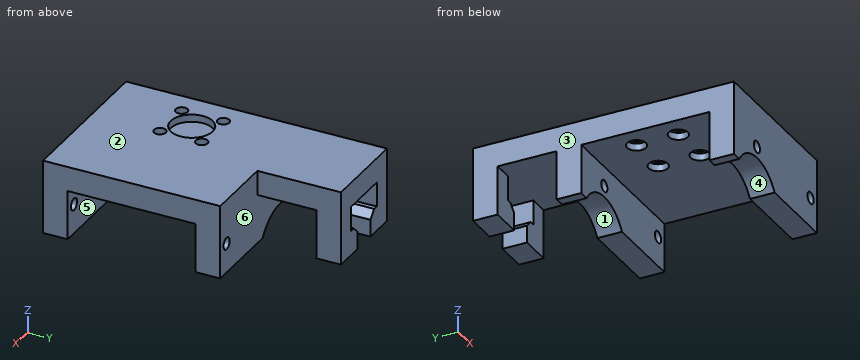
```python
from build123d import *

# Parameters (mm, degrees)
SKETCH_1_W                   = 32.5
SKETCH_1_H                   = 36
EXTRUDE_1_DEPTH              = 15
SKETCH_2_W                   = 10
SKETCH_2_H                   = 26
CUT_EXTRUDE_1_DEPTH          = 41.065571255
HOLE_WIZARD_M2_1_D           = 2.4
HOLE_WIZARD_M2_1_DEPTH       = 5
CUT_EXTRUDE_3_DEPTH          = 39.079686186
CUT_EXTRUDE_3_DEPTH_BACK     = 39.079686186
SKETCH_4_R                   = 8.25
SKETCH_4_R_2                 = 1.2
HOLE_WIZARD_M2_2_D           = 2.4
HOLE_WIZARD_M2_2_CBORE_D     = 3.85
HOLE_WIZARD_M2_2_CBORE_DEPTH = 1.45
SKETCH_13_W                  = 18
SKETCH_13_H                  = 15
EXTRUDE_3_DEPTH              = 17
CUT_EXTRUDE_4_DEPTH          = 42.401237904
CUT_EXTRUDE_4_DEPTH_BACK     = 10
SKETCH_14_W                  = 18
SKETCH_14_H                  = 12
CUT_EXTRUDE_5_REACH          = 59.429
SKETCH_15_W                  = 5
SKETCH_15_H                  = 10
CUT_EXTRUDE_START            = -5
SKETCH_16_W                  = 10
SKETCH_16_H                  = 5
CUT_EXTRUDE_6_DEPTH          = 5
CHAMFER_1_SIZE               = 1.5
CUT_EXTRUDE_7_DEPTH          = 1.5


with BuildPart() as part:
    # ｽｹｯﾁ1 → ﾎﾞｽ - 押し出し1 (new body)
    with BuildSketch(Plane.XY):
        Rectangle(SKETCH_1_W, SKETCH_1_H)
    extrude(amount=EXTRUDE_1_DEPTH)

    # ｽｹｯﾁ2 → ｶｯﾄ - 押し出し1 (cut, through all)
    with BuildSketch(Plane(origin=(16.25, 0, 0), x_dir=(0, 0, -1), z_dir=(1, 0, 0))):
        with Locations((-5, 0)):
            Rectangle(SKETCH_2_W, SKETCH_2_H)
    extrude(amount=-CUT_EXTRUDE_1_DEPTH, mode=Mode.SUBTRACT)

    # M2 すきま穴1
    with Locations(Plane.XZ.offset(-13)):
        with Locations((13.75, 6), (-7.25, 6)):
            hole_wizard_m2_1 = Hole(HOLE_WIZARD_M2_1_D / 2, depth=HOLE_WIZARD_M2_1_DEPTH)

    # ｽｹｯﾁ4 → ｶｯﾄ - 押し出し3 (cut, two sides: drawn at the far end of the back side and taken through both)
    with BuildSketch(Plane.XZ.offset(-13).offset(-CUT_EXTRUDE_3_DEPTH_BACK)):
        with Locations((-7.25, -4.5)):
            Circle(SKETCH_4_R)
        with Locations(Location((-7.25, 6, 0), (0, 0, 270))):
            Circle(SKETCH_4_R_2)
    extrude(amount=CUT_EXTRUDE_3_DEPTH + CUT_EXTRUDE_3_DEPTH_BACK, mode=Mode.SUBTRACT)

    # ﾐﾗｰ1: M2 すきま穴1 across plane
    add(hole_wizard_m2_1.mirror(Plane.ZX), mode=Mode.SUBTRACT)

    # M2 丸平ねじ用座ぐり穴2 (through all)
    with Locations(Plane(origin=(0, 0, 10), x_dir=(-1, 0, 0), z_dir=(0, 0, -1))):
        with Locations((11.492640687, 4.242640687), (3.007359313, -4.242640687), (11.492640687, -4.242640687), (3.007359313, 4.242640687)):
            CounterBoreHole(HOLE_WIZARD_M2_2_D / 2, HOLE_WIZARD_M2_2_CBORE_D / 2, HOLE_WIZARD_M2_2_CBORE_DEPTH)

    # ｽｹｯﾁ13 → ﾎﾞｽ - 押し出し3 (add)
    with BuildSketch(Plane(origin=(0, 18, 0), x_dir=(1, 0, 0), z_dir=(0, 1, 0))):
        with Locations((-7.25, -7.5)):
            Rectangle(SKETCH_13_W, SKETCH_13_H)
    extrude(amount=EXTRUDE_3_DEPTH)

    # ｽｹｯﾁ14 → ｶｯﾄ - 押し出し4 (cut, two sides: drawn at the far end of the back side and taken through both)
    with BuildSketch(Plane(origin=(0, 0, 0), x_dir=(-1, 0, 0), z_dir=(0, 0, -1)).offset(-CUT_EXTRUDE_4_DEPTH_BACK)):
        with Locations((7.25, 24)):
            Rectangle(SKETCH_14_W, SKETCH_14_H)
    extrude(amount=CUT_EXTRUDE_4_DEPTH + CUT_EXTRUDE_4_DEPTH_BACK, mode=Mode.SUBTRACT)

    # ｽｹｯﾁ15 → ｶｯﾄ - 押し出し5 (cut, up to next)
    with BuildSketch(Plane(origin=(0, 35, 0), x_dir=(1, 0, 0), z_dir=(0, 1, 0)), mode=Mode.PRIVATE) as cut_extrude_5_sk1:
        with Locations((-7.25, -5)):
            Rectangle(SKETCH_15_W, SKETCH_15_H)
    cut_extrude_5_tool1 = extrude(cut_extrude_5_sk1.sketch, amount=-CUT_EXTRUDE_5_REACH, mode=Mode.PRIVATE) & part.part
    add(cut_extrude_5_tool1.solids().sort_by_distance((-7.25, 35, 5))[0], mode=Mode.SUBTRACT)

    # ｽｹｯﾁ16 → ｶｯﾄ - 押し出し6 (cut)
    with BuildSketch(Plane(origin=(0, 35, 0), x_dir=(1, 0, 0), z_dir=(0, 1, 0)).offset(CUT_EXTRUDE_START)):
        with Locations((-7.25, -7.5)):
            Rectangle(SKETCH_16_W, SKETCH_16_H)
    extrude(amount=CUT_EXTRUDE_6_DEPTH, mode=Mode.SUBTRACT)

    # 面取り1
    chamfer_1_edges = [part.edges().sort_by_distance(p)[0] for p in [
        (-9.75, 32.5, 5),
        (-4.75, 32.5, 5),
    ]]
    chamfer(chamfer_1_edges, length=CHAMFER_1_SIZE)

    # ｽｹｯﾁ17 → ｶｯﾄ - 押し出し7 (cut)
    with BuildSketch(Plane.XY.offset(15)):
        with BuildLine():
            Line((-7, 4.242640687), (-7.5, 4.242640687))
            ThreePointArc((-7.5, 4.242640687), (-10.25520382, -3.00520382), (-3.007359313, -0.25))
            Line((-3.007359313, -0.25), (-3.007359313, 0.25))
            ThreePointArc((-3.007359313, 0.25), (-4.24479618, 3.00520382), (-7, 4.242640687))
        make_face()
    extrude(amount=-CUT_EXTRUDE_7_DEPTH, mode=Mode.SUBTRACT)


solid = part.part
```
Design review of the part built by this model. Coordinates are the model's own, in mm. Face numbers are marked on the shaded views. A direction names the side the tool comes from. Coordinates: 2 decimals unless noted, no trailing zeros. Write each loop counter-clockwise with the first axis right and the second up, starting at its lowest first coordinate (ties: lowest second). Pieces come first, ordered by that corner, then holes.
1) Add section C-C (z = 8.75). Write out the cut boundary in (x, y).
2) Machinability: for the marked faces 4, 5 and 6, which of the approach directions +Z, -Z, +X, -X, +Y, -Y give a long, thin tool a straight path to every point of the face, cutting with its end or side? Answer none if there is none.
3) Add section B-B (x = 13.75). Write out the cut boundary in (y, z), plus the area to 3 significant figures.
4) To check wall thickness, follow L1, parallel to Y at x = 0, z = 3.5; L2, parallel to X at y = -15.85, z = 6; L3, parallel to Z at x = -7.25, y = 16.2. State the ranges of each line that lie inside material, in increasing order.
5) Mouldability with a two-part tool opening along X and no side actions: class the marked faces 1, 2 and 3 as +X half, -X half, draft (parallel to the pull), parting line (faces both ways), or undercut.
6) Insertion check: pin 1 (2 mm diameter, centred on x = -11.49, y = -4.24, fed in from -Z) (3 decimals); pin 2 (12 mm diameter, centred on x = 10.5, y = 3, fed in from -Z); pin 3 (3 mm diameter, centred on x = -11.49, y = 4.24, fed in from -Z); pin 4 (4 mm diameter, centred on y = 33, z = 2.5, fed in from +X). Each pin has a flat end and moves straight along its axis. Give the tip position at first contact, or say it passes through.
7) Add section D-D (y = 9.5). Write out the cut boundary in (x, z), plus the area to 4 significant figures.
8) Add section A-A (z = 6). State how many separate pieces and enclosed holes the cut face has, plus the area to 3 significant figures.
Check result:
1. outline: (-16.25, -18) - (16.25, -18) - (16.25, -13) - (-16.25, -13) - close; (-16.25, 13) - (16.25, 13) - (16.25, 18) - (-16.25, 18) - close; (-16.25, 30) - (-12.25, 30) - (-12.25, 35) - (-16.25, 35) - close; (-2.25, 30) - (1.75, 30) - (1.75, 35) - (-2.25, 35) - close
2. face 4: -Z, -Y
2. face 5: -Z, +X, -X
2. face 6: -Z, +X
3. outline: (-18, 0) - (-13, 0) - (-13, 4.8) - (-18, 4.8) - close; (-18, 7.2) - (-13, 7.2) - (-13, 10) - (13, 10) - (13, 7.2) - (18, 7.2) - (18, 15) - (-18, 15) - close; (13, 0) - (18, 0) - (18, 4.8) - (13, 4.8) - close
3. area: 256 mm2
4. L1: y = -18 to -13, 13 to 18, 30 to 35
4. L2: x = -16.25 to -8.45, -6.05 to 12.55, 14.95 to 16.25
4. L3: z = 3.75 to 4.8, 7.2 to 15
5. face 1: undercut
5. face 2: draft
5. face 3: -X half
6. pin 1: passes through
6. pin 2: stops at z = 10
6. pin 3: stops at z = 11.45
6. pin 4: stops at x = 1.75
7. outline: (-16.25, 10) - (16.25, 10) - (16.25, 15) - (-16.25, 15) - close
7. area: 162.5 mm2
8. separate pieces: 8
8. enclosed holes: 0
8. area: 317 mm2
